Here's how the part is built. I have some questions about the finished solid (model axes, mm). Face numbers are marked on the shaded views. A direction names the side the tool comes from. Give positions to 0.01 mm unless a question says otherwise; leave off trailing zeros. Loops run counter-clockwise (first coordinate to the right, second up) from the corner with the lowest first, then second, coordinate; pieces in that order, holes last.
Q1. I need wall thicknesses on line 1 (X direction, y = 0, z = 7.75); line 2 (Y direction, x = 14, z = 16); line 3 (X direction, y = 0.75, z = 8). Which ranges of each line are inside material? Lowest first, please.
Q2. If we section it at B-B (y = 0): Please give me the cut outline in (x, z).
Q3. For the marked faces 1, 2 and 3, which set-ups out of +Z, -Z, +X, -X, +Y, -Y let a thin tool reach every point of the face, with its end or its side?
Q4. If we section it at A-A (z = 17): Please give me the cut outline in (x, y) (1 decimal).
Q5. We'd pull the mould along X, two halves only. Please class the marked faces 4, 5 and 6: +X half, -X half, draft (parallel to the pull), parting line (faces both ways), or undercut.
Q6. If we section it at C-C (x = -13): Please give me the cut outline in (y, z).
Q7. Will these pins go through, and if not, where does the flat tip stop? P1, Ø3, axis at x = 14, y = 0, coming from the +Z side; P2, Ø5, axis at x = -14, y = 0, coming from the -Z side; P3, Ø1.5, axis at x = 6, y = 3.5, coming from the +Z side; P4, Ø1.5, axis at x = -3, y = 3, coming from the +Z side.
Autodesk Inventor part; units mm, degrees
ref_plane "YZ Plane" through (0, 0, 0) normal (1, 0, 0) x (0, 1, 0)
ref_plane "XZ Plane" through (0, 0, 0) normal (0, 1, 0) x (-1, 0, 0)
ref_plane "XY Plane" through (0, 0, 0) normal (0, 0, 1) x (1, 0, 0)
sketch "Sketch1" plane through (0, 0, 0) normal (0, 0, 1) x (1, 0, 0)
  circle A0 centre (-14, 0) radius 1.8875
  circle A1 centre (-14, 0) radius 5
  line L0 (0, -7) -> (0, 7)
  circle A2 centre (14, 0) radius 1.8875
  circle A3 centre (14, 0) radius 5
  line L1 (-14, 5) -> (-5, 5)
  line L2 (-5, 5) -> (0, 5)
  line L3 (14, 5) -> (5, 5)
  line L4 (5, 5) -> (0, 5)
  line L5 (-26.6, 0) -> (26.6, 0)
  line L6 (-14, -5) -> (-5, -5)
  line L7 (-5, -5) -> (0, -5)
  line L8 (5, -5) -> (0, -5)
  line L9 (14, -5) -> (5, -5)
  point P0 (0, 0)
  point P1 (14, 5)
  point P2 (-14, -5)
  point P3 (14, -5)
  dimension "d1" = 10
  dimension "d0" = 3.775
  dimension "d2" = 28
  dimension "d3" = 5
  dimension "d4" = 5
extrude "Extrusion1" add sketch "Sketch1" along normal blind 25 contours L5 A1 A0 | A0 L5 A1 | L5 L0 L7 L6 A1 | A1 L1 L2 L0 L5 | L5 A3 L9 L8 L0 | L0 L4 L3 A3 L5 | L5 A2 A3 | A3 L5 A2
sketch "Sketch2" plane through (-14, 5, 0) normal (0, 1, 0) x (1, 0, 0)
  line L0 (28, -25) -> (0, -25)
  line L1 (4, -25) -> (9, -20)
  line L2 (9, -20) -> (14, -20)
  line L3 (28, 0) -> (0, 0)
  line L4 (28, 0) -> (28, -25)
  line L5 (28, -12.5) -> (1.8875, -12.5)
  line L6 (1.8875, -25) -> (1.8875, 0)
  line L7 (28, 0) -> (0, 0)
  line L8 (4, 0) -> (9, -5)
  line L9 (9, -5) -> (14, -5)
  line L10 (14, -25) -> (14, 0)
  line L11 (24, -25) -> (19, -20)
  line L12 (19, -20) -> (14, -20)
  line L13 (24, 0) -> (19, -5)
  line L14 (19, -5) -> (14, -5)
  point P0 (14, 0)
  point P1 (4, 0)
  dimension "d7" = 45
  dimension "d8" = 15
  dimension "d9" = 10
extrude "Extrusion2" cut sketch "Sketch2" against normal up to surface (10 mm away) contours L0 L10 L12 L11 | L0 L1 L2 L10 | L13 L14 L10 L3 | L9 L8 L3 L10
fillet "Fillet1" radius 1 20 edges at (-12, -5, 25) (-12, 5, 25) (-19, 0, 25) (-7.5, 5, 22.5) (0, 5, 20) (7.5, 5, 22.5) (19, 0, 25) (-7.5, -5, 22.5) (0, -5, 20) (7.5, -5, 22.5) (19, 0, 0) (-12, 5, 0) (-12, -5, 0) (7.5, -5, 2.5) (0, -5, 5) (-7.5, -5, 2.5) (-19, 0, 0) (-7.5, 5, 2.5) (0, 5, 5) (7.5, 5, 2.5)
properties part number "ConectorBrazos"
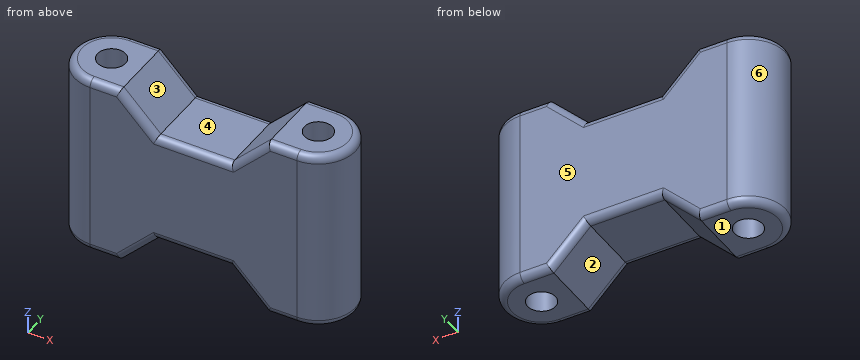
Check sheet entries:
1. line 1: x = -19 to -15.89, -12.11 to 12.11, 15.89 to 19
1. line 2: y = -5 to -1.89, 1.89 to 5
1. line 3: x = -18.94 to -15.73, -12.27 to 12.27, 15.73 to 18.94
2. outline: (-19, 1) arc R1 ccw to (-18, 0) - (-15.89, 0) - (-15.89, 25) - (-18, 25) arc R1 ccw to (-19, 24) - close; (-12.11, 0) - (-10, 0) - (-5, 5) - (5, 5) - (10, 0) - (12.11, 0) - (12.11, 25) - (10, 25) - (5, 20) - (-5, 20) - (-10, 25) - (-12.11, 25) - close; (15.89, 0) - (18, 0) arc R1 ccw to (19, 1) - (19, 24) arc R1 ccw to (18, 25) - (15.89, 25) - close
3. face 1: -Z, +X, -X, +Y, -Y
3. face 2: -Z, +Y, -Y
3. face 3: +Z, +Y, -Y
4. outline: (-14, -5) - (14, -5) arc R5 ccw to (14, 5) - (-14, 5) arc R5 ccw to start; hole circle Ø3.8 at (-14, 0); hole circle Ø3.8 at (14, 0)
5. face 4: undercut
5. face 5: draft
5. face 6: -X half
6. outline: (-5, 1) arc R1 ccw to (-4, 0) - (-1.6, 0) - (-1.6, 25) - (-4, 25) arc R1 ccw to (-5, 24) - close; (1.6, 0) - (4, 0) arc R1 ccw to (5, 1) - (5, 24) arc R1 ccw to (4, 25) - (1.6, 25) - close
7. P1: passes through
7. P2: stops at z = 0
7. P3: stops at z = 21.75
7. P4: stops at z = 20
